Part model, mm, in its own coordinate system. Face numbers are marked on the shaded views. A direction names the side the tool comes from. Coordinates: 2 decimals unless noted, no trailing zeros. Loops run counter-clockwise (first coordinate to the right, second up) from the corner with the lowest first, then second, coordinate; pieces in that order, holes last. Notation, with made-up numbers: (28.25, 88) -> (81.25, 88) arc R16 cw to (81.25, 114) -> close; hole circle Ø1 at (41.5, 33.5). An arc over 180 degrees is marked (long way). Use one line per item in the form item = value. Start each with the question number.
(1) Pin check, flat tips, straight feed: P1, Ø6, axis at x = -19.5, z = 49.5, coming from the -Y side; P2, Ø3, axis at y = -80, z = 60.5, coming from the -X side; P3, Ø3, axis at y = -73, z = 39, coming from the +X side. Stop position of each tip, or through.
(2) Band-saw the part on B-B on x = -2. Give the cut face in (y, z), then the cut area to 3 significant figures.
(3) 3-axis set-ups, long thin cutter, end or side, ignore diameter. For the marked faces 4, 5 and 6: which of +Z, -Z, +X, -X, +Y, -Y reach the whole face in a straight line?
(4) Band-saw the part on D-D on y = -76.5. Give the cut face in (x, z).
(5) Band-saw the part on C-C on x = 29. Give the cut face in (y, z), then the cut area to 3 significant figures.
(6) Mould opens along X. For the marked faces 1, 2 and 3 say: +X half, -X half, draft (parallel to the pull), parting line (faces both ways), or undercut.
(7) Drill centre lines: L1, parallel to Y at x = 33, z = 60; L2, parallel to X at y = -115, z = 29; L3, parallel to X at y = -78, z = 20.5. Where is each one in solid material? Low to high. Write a range as [from, to].
(8) Band-saw the part on A-A on y = -100. Give the cut face in (x, z), then the cut area to 3 significant figures.
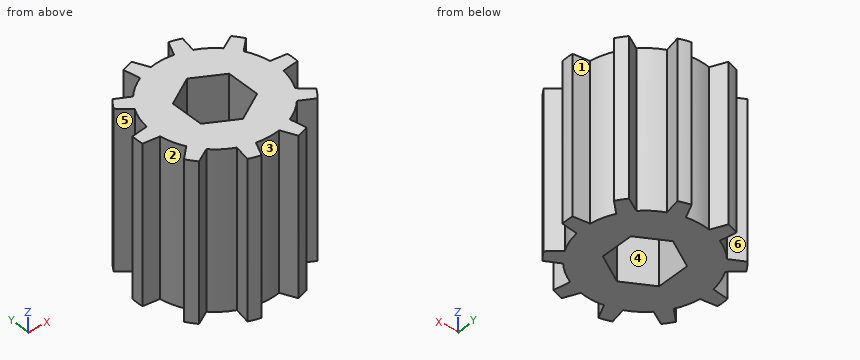
```python
from build123d import *

# Parameters (mm, degrees)
SKETCH011_R           = 31.75
PAD009_DEPTH          = 80.15
PAD010_DEPTH          = 80.15
POLARPATTERN006_COUNT = 10
POCKET010_DEPTH       = 80.151


with BuildPart() as part:
    # Sketch011 → Pad009 (new body)
    with BuildSketch(Plane.XY):
        Circle(SKETCH011_R)
    extrude(amount=PAD009_DEPTH)

    # Sketch009 → Pad010 (join)
    with BuildSketch(Plane.XY):
        with BuildLine():
            ThreePointArc((39.636631, -3), (39.75, 0), (39.636631, 3))
            Line((31.497024, 4), (39.636631, 3))
            Line((31.497024, 4), (21.166667, 0))
            Line((21.166667, 0), (31.497024, -4))
            Line((31.497024, -4), (39.636631, -3))
        make_face()
    pad010 = extrude(amount=PAD010_DEPTH)

    # PolarPattern006: Pad010 ×10 about axis
    polarpattern006_axis = Axis((0, 0, 0), (0, 0, 1))
    for i in range(1, POLARPATTERN006_COUNT):
        add(pad010.rotate(polarpattern006_axis, i * 360 / POLARPATTERN006_COUNT))

    # Sketch010 → Pocket010 (cut, through all)
    with BuildSketch(Plane.XY):
        Polygon((14.3875, 8.306627), (0, 16.613254), (-14.3875, 8.306627), (-14.3875, -8.306627), (0, -16.613254), (14.3875, -8.306627), align=None)
    extrude(amount=POCKET010_DEPTH, mode=Mode.SUBTRACT)


with BuildPart() as part_1:
    # Body024 placement: moved
    add(part.part.moved(Location((0, -100, 0))))


solid = part_1.part
```
A:
q1.P1 = -127.13
q1.P2 = -33.83
q1.P3 = 30.49
q2.outline = (-131.69, 0) -> (-115.46, 0) -> (-115.46, 80.15) -> (-131.69, 80.15) -> close; (-84.54, 0) -> (-68.31, 0) -> (-68.31, 80.15) -> (-84.54, 80.15) -> close
q2.area = 2,600 mm²
q3.face_4 = +Z, -Z
q3.face_5 = +Z, -Z, -X
q3.face_6 = +Z, -Z, +Y
q4.outline = (-32.06, 0) -> (-26.29, 0) -> (-26.29, 80.15) -> (-32.06, 80.15) -> close; (-21.35, 0) -> (21.35, 0) -> (21.35, 80.15) -> (-21.35, 80.15) -> close; (26.29, 0) -> (32.06, 0) -> (32.06, 80.15) -> (26.29, 80.15) -> close
q5.outline = (-125, 0) -> (-116.37, 0) -> (-116.37, 80.15) -> (-125, 80.15) -> close; (-112.93, 0) -> (-87.07, 0) -> (-87.07, 80.15) -> (-112.93, 80.15) -> close; (-83.63, 0) -> (-75, 0) -> (-75, 80.15) -> (-83.63, 80.15) -> close
q5.area = 3,460 mm²
q6.face_1 = +X half
q6.face_2 = -X half
q6.face_3 = undercut
q7.L1 = [-122.16, -120.1], [-103.82, -96.18], [-79.9, -77.84]
q7.L2 = [-27.98, -2.79], [2.79, 27.98]
q7.L3 = [-33.11, -23.58], [-22.89, 22.89], [23.58, 33.11]
q8.outline = (-39.75, 0) -> (-14.39, 0) -> (-14.39, 80.15) -> (-39.75, 80.15) -> close; (14.39, 0) -> (39.75, 0) -> (39.75, 80.15) -> (14.39, 80.15) -> close
q8.area = 4,070 mm²
